Autodesk Inventor part; units mm, degrees
ref_plane "YZ Plane" through (0, 0, 0) normal (1, 0, 0) x (0, 1, 0)
ref_plane "XZ Plane" through (0, 0, 0) normal (0, 1, 0) x (-1, 0, 0)
ref_plane "XY Plane" through (0, 0, 0) normal (0, 0, 1) x (1, 0, 0)
sketch "Sketch1" plane through (0, 0, 0) normal (0, 0, 1) x (1, 0, 0)
  line L0 (-71.8432, 70.6031) -> (131.3568, 70.6031)
  line L1 (131.3568, -742.1969) -> (-71.8432, -742.1969)
  line L2 (-71.8432, -742.1969) -> (-71.8432, 70.6031)
  line L3 (131.3568, -132.5969) -> (-10.9328, -162.8415)
  line L4 (131.3568, -165.0562) -> (-19.8283, -197.1916)
  arc A0 (-24.3438, -165.6921) -> (-17.7426, -196.7483) centre (-21.0432, -181.2202) ccw
  line L5 (131.3568, 70.6031) -> (131.3568, -132.5969)
  line L6 (131.3568, -165.0562) -> (131.3568, -742.1969) construction
  line L7 (131.3568, -386.5969) -> (-10.9328, -416.8415)
  line L8 (131.3568, -419.0562) -> (-19.8283, -451.1916)
  arc A1 (-24.3438, -419.6921) -> (-17.7426, -450.7483) centre (-21.0432, -435.2202) ccw
  line L9 (131.3568, -640.5969) -> (-10.9328, -670.8415)
  line L10 (131.3568, -673.0562) -> (-19.8283, -705.1916)
  arc A2 (-24.3438, -673.6921) -> (-17.7426, -704.7483) centre (-21.0432, -689.2202) ccw
  line L11 (131.3568, -165.0562) -> (131.3568, -386.5969)
  line L12 (131.3568, -419.0562) -> (131.3568, -640.5969)
  line L13 (131.3568, -673.0562) -> (131.3568, -742.1969)
  line L14 (-24.3438, -165.6921) -> (-10.9328, -162.8415)
  line L15 (-24.3438, -419.6921) -> (-10.9328, -416.8415)
  line L16 (-24.3438, -673.6921) -> (-9.6152, -670.5614)
  point P0 (0, 0)
  dimension "d0" = 203.2
  dimension "d1" = 812.8
  dimension "d3" = 31.75
  dimension "d4" = 203.2
  dimension "d7" = 254
  dimension "d48" = 152.4
extrude "Extrusion1" add sketch "Sketch1" along normal blind 18.796
sketch "Sketch3" plane through (0, 0, 18.796) normal (0, 0, 1) x (1, 0, 0)
  line L0 (-71.8432, 70.6031) -> (131.3568, 70.6031)
  line L1 (4.3568, 70.6031) -> (55.5231, 70.6031)
  line L2 (55.5231, 70.6031) -> (55.5231, 51.8071)
  line L3 (55.5231, 51.8071) -> (4.3568, 51.8071)
  line L4 (4.3568, 51.8071) -> (4.3568, 70.6031)
  line L5 (-71.8432, 70.6031) -> (-71.8432, -742.1969)
  point P0 (0, 0)
  dimension "d31" = 18.796
  dimension "d32" = 0
  dimension "d34" = 76.2
extrude "Extrusion2" cut sketch "Sketch3" against normal blind 18.796
sketch "Sketch5" plane through (0, 0, 18.796) normal (0, 0, 1) x (1, 0, 0)
  line L0 (80.5568, -81.7969) -> (105.9568, -81.7969)
  line L1 (105.9568, -81.7969) -> (105.9568, -100.5929)
  line L2 (105.9568, -100.5929) -> (80.5568, -100.5929)
  line L3 (80.5568, -100.5929) -> (80.5568, -81.7969)
  line L4 (-71.8432, 70.6031) -> (-71.8432, -742.1969)
  line L5 (131.3568, -132.5969) -> (131.3568, 70.6031)
  line L6 (131.3568, 70.6031) -> (55.5231, 70.6031)
  line L7 (-21.0432, -81.7969) -> (-46.4432, -81.7969)
  line L8 (-46.4432, -81.7969) -> (-46.4432, -100.5929)
  line L9 (-46.4432, -100.5929) -> (-21.0432, -100.5929)
  line L10 (-21.0432, -100.5929) -> (-21.0432, -81.7969)
  line L11 (4.3568, -742.1969) -> (55.1568, -742.1969)
  line L12 (55.1568, -742.1969) -> (55.1568, -723.4009)
  line L13 (55.1568, -723.4009) -> (4.3568, -723.4009)
  line L14 (4.3568, -723.4009) -> (4.3568, -742.1969)
  line L15 (-71.8432, -742.1969) -> (131.3568, -742.1969)
  point P0 (0, 0)
  dimension "d51" = 25.4
  dimension "d52" = 18.796
  dimension "d53" = 25.4
  dimension "d54" = 152.4
  dimension "d55" = 25.4
  dimension "d56" = 18.796
  dimension "d57" = 25.4
  dimension "d58" = 50.8
  dimension "d59" = 18.796
  dimension "d60" = 0
  dimension "d61" = 76.2
extrude "Extrusion4" cut sketch "Sketch5" against normal blind 25.4
sketch "Sketch6" plane through (0, 0, 18.796) normal (0, 0, 1) x (1, 0, 0)
  line L0 (-71.8432, 70.6031) -> (4.3568, 70.6031)
  line L1 (-71.8432, 1.0071) -> (-53.0472, 1.0071)
  line L2 (-71.8432, -30.9969) -> (-53.0472, -30.9969)
  line L3 (-71.8432, 1.0071) -> (-71.8432, -30.9969)
  line L4 (-71.8432, -742.1969) -> (-71.8432, 70.6031)
  line L5 (-53.0472, 1.0071) -> (-53.0472, -30.9969)
  point P0 (0, 0)
  dimension "d66" = 32.004
  dimension "d68" = 18.796
extrude "Extrusion5" cut sketch "Sketch6" against normal blind 25.4
sketch "Sketch8" plane through (0, 0, 18.796) normal (0, 0, 1) x (1, 0, 0)
  line L0 (4.3568, -742.1969) -> (4.3568, -723.4009)
  line L1 (4.3568, -723.4009) -> (55.1568, -723.4009)
  point P0 (0, 0)
  point P1 (4.3568, 51.8071)
  point P2 (55.5513, 51.8071)
hole "Hole2" at (4.3568, 51.8071, 18.796) at (55.5513, 51.8071, 18.796) at (4.3568, -723.4009, 18.796) at (55.1568, -723.4009, 18.796) direction (0, 0, -1) diameter 6.35 end through all
sketch "Sketch9" plane through (0, 0, 18.796) normal (0, 0, 1) x (1, 0, 0)
  line L0 (-21.0432, -81.7969) -> (-46.4432, -81.7969)
  line L1 (-21.0432, -100.5929) -> (-21.0432, -81.7969)
  line L2 (-46.4432, -100.5929) -> (-21.0432, -100.5929)
  line L3 (105.9568, -81.7969) -> (80.5568, -81.7969)
  line L4 (80.5568, -100.5929) -> (105.9568, -100.5929)
  line L5 (105.9568, -100.5929) -> (105.9568, -81.7969)
  point P0 (0, 0)
  point P1 (-46.6954, -81.6809)
hole "Hole3" at (-46.6954, -81.6809, 18.796) at (-21.0432, -81.7969, 18.796) at (-21.0432, -100.5929, 18.796) at (-46.4432, -100.5929, 18.796) at (80.5568, -81.7969, 18.796) at (80.5568, -100.5929, 18.796) at (105.9568, -100.5929, 18.796) at (105.9568, -81.7969, 18.796) direction (0, 0, -1) diameter 6.35 end through all
sketch "Sketch10" plane through (0, 0, 18.796) normal (0, 0, 1) x (1, 0, 0)
  line L0 (-53.0472, 1.0071) -> (-71.8432, 1.0071)
  point P0 (0, 0)
  point P1 (-53.0472, -31.6336)
hole "Hole4" at (-53.0472, 1.0071, 18.796) at (-53.0472, -31.6336, 18.796) direction (0, 0, -1) diameter 6.35 end through all
sketch "Sketch11" plane through (0, 0, 18.796) normal (0, 0, 1) x (1, 0, 0)
  line L0 (-71.8432, -30.9969) -> (-71.8432, -742.1969)
  line L1 (55.1568, -726.5759) -> (55.1568, -742.1969)
  line L2 (131.3568, -742.1969) -> (131.3568, -673.0562)
  point P0 (0, 0)
  point P1 (29.7568, -91.1319)
  point P2 (-33.7432, -732.2316)
  point P3 (55.1568, -734.3864)
  point P4 (93.2568, -734.3864)
  dimension "d92" = 101.6
  dimension "d93" = 38.1
  dimension "d94" = 38.1
hole "Hole5" at (29.7568, -91.1319, 18.796) at (-33.7432, -732.2316, 18.796) at (55.1568, -734.3864, 18.796) at (93.2568, -734.3864, 18.796) direction (0, 0, -1) diameter 6.35 end through all
properties part number "rack sides" material "Wood (Birch)"
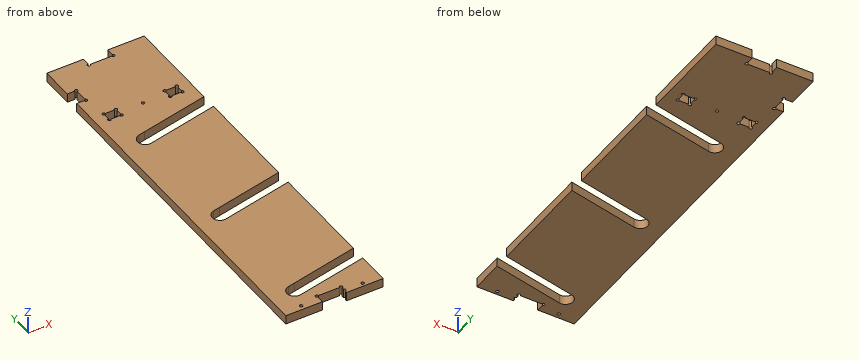
Here's how the part is built. I have some questions about the finished solid (model axes, mm). Round coordinates to 2 decimals unless told otherwise and drop trailing zeros. Loops run counter-clockwise (first coordinate to the right, second up) from the corner with the lowest first, then second, coordinate; pieces in that order, holes last.
1. If we section it at B-B on z = 4.75: Count the separate pieces of the cut face and the enclosed holes in it, plus the area to 3 significant figures.
Answer list:
separate pieces: 1
enclosed holes: 5
area: 145,000 mm2
2. If I drill on line 1 along Y through (x, z) = (105, 12); line 2 along Y through (x, z) = (-33.5, 15); line 3 along Y through (x, z) = (109.5, 14.5), over which ranges is the centre line in solid material (lowest first)?
Answer list:
line 1: y = -742.2 to -678.66, -646.2 to -424.66, -392.2 to -170.66, -138.2 to -103.62, -78.77 to 70.6
line 2: y = -742.2 to -735.4, -729.07 to -699.06, -679.38 to -445.06, -425.38 to -191.06, -171.38 to -100.59, -81.8 to 70.6
line 3: y = -742.2 to -677.7, -645.24 to -423.7, -391.24 to -169.7, -137.24 to 70.6
3. For P1, Ø5, axis at x = 105.96, y = -81.8, coming from the -Z side; P2, Ø1.5, axis at y = -28.5, z = 15.5, coming from the -X side; P3, Ø8.5, axis at x = 80.56, y = -81.8, coming from the +Z side; P4, Ø6, axis at x = 28.5, z = 14.5, coming from the -Y side, each with a flat end and sliding along its axis, tell me the tip position at first contact or that it passes through.
Answer list:
P1: passes through
P2: stops at x = -53.05
P3: stops at z = 18.8
P4: stops at y = -723.4
4. If we section it at A-A on x = 117: Write out the boundary of the cut face in (y, z), plus the area to 3 significant figures.
Answer list:
outline: (-742.2, 0) - (-676.11, 0) - (-676.11, 18.8) - (-742.2, 18.8) - close; (-643.65, 0) - (-422.11, 0) - (-422.11, 18.8) - (-643.65, 18.8) - close; (-389.65, 0) - (-168.11, 0) - (-168.11, 18.8) - (-389.65, 18.8) - close; (-135.65, 0) - (70.6, 0) - (70.6, 18.8) - (-135.65, 18.8) - close
area: 13,400 mm2
